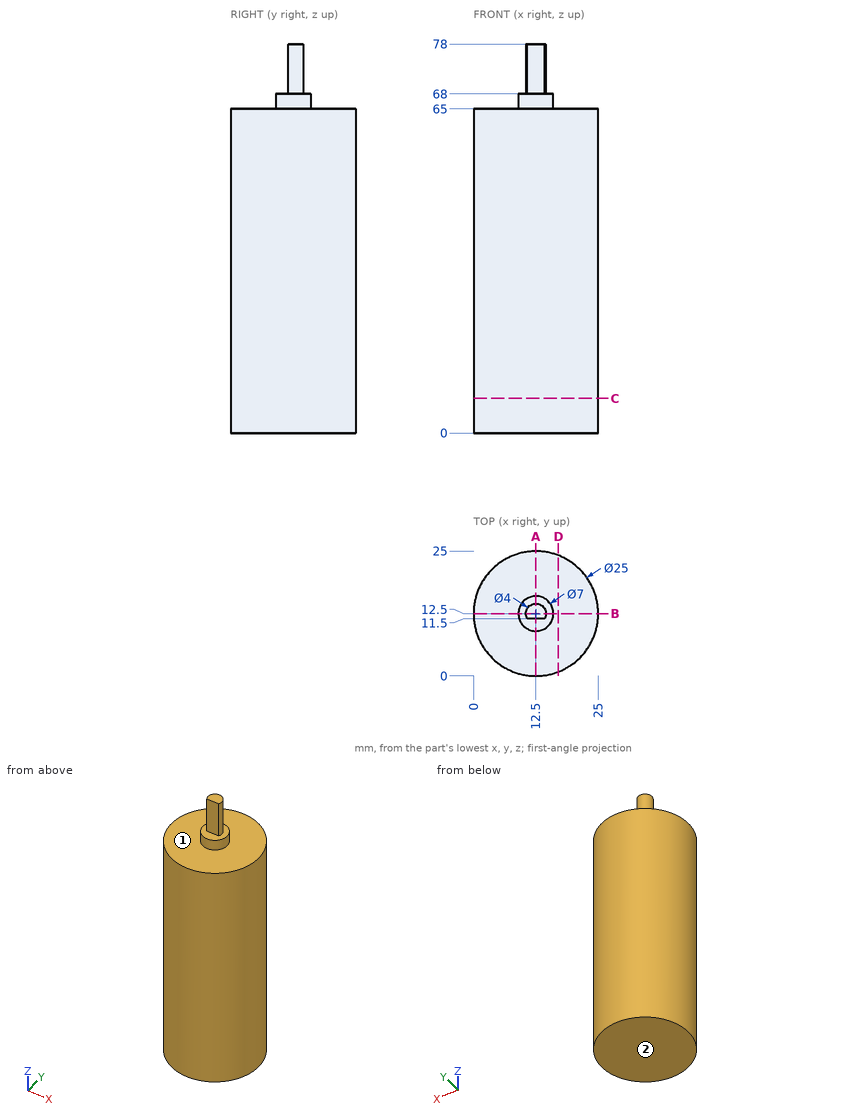
Answer from the drawing. Dimensions are ordinates in mm from the lowest x, y and z of the part. A direction names the side the tool comes from. Give positions to 0.01 mm unless a question says otherwise; leave off trailing zeros. Order: outer loops, then holes, each group sorted by start corner. A loop starts at its lowest first (then second) coordinate and runs counter-clockwise, first axis right, second up.
(1) Given pin 1 (1 mm diameter, centred on x = 13, z = 75.5, fed in from -Y); pin 2 (1.5 mm diameter, centred on y = 14, z = 22, fed in from -X); pin 3 (1 mm diameter, centred on x = 20.5, y = 3.5, fed in from +Z), each flat-ended and moving along its own axis, determine where each tip first touches the part or whether it passes through.
(2) For the marked faces 1 and 2, determine the directions among +Z, -Z, +X, -X, +Y, -Y from which every point of the face is accessible in a straight line to the end or side of a thin tool.
(3) Find section A-A (x = 12.5). Give the vertices of the cut face in (y, z).
(4) Find section B-B (y = 12.5). Give the vertices of the cut face in (x, z), plus the area to 3 significant figures.
(5) Find section C-C (z = 7). Give the vertices of the cut face in (x, y), plus the area to 3 significant figures.
(6) Straight lines are drawn through the part: L1, parallel to Z at x = 12, y = 23.25; L2, parallel to Y at x = 12, z = 45.5; L3, parallel to X at y = 3.5, z = 28.5 (1 decimal). For each, find the intervals that lie inside material, in ascending order.
(7) Find section D-D (x = 17). Give the vertices of the cut face in (y, z).
Result sheet:
1. pin 1: stops at y = 11.5
1. pin 2: stops at x = 0.02
1. pin 3: stops at z = 65
2. face 1: +Z
2. face 2: -Z, +X, -X, +Y, -Y
3. outline: (0, 0) - (25, 0) - (25, 65) - (16, 65) - (16, 68) - (14.5, 68) - (14.5, 78) - (11.5, 78) - (11.5, 68) - (9, 68) - (9, 65) - (0, 65) - close
4. outline: (0, 0) - (25, 0) - (25, 65) - (16, 65) - (16, 68) - (14.5, 68) - (14.5, 78) - (10.5, 78) - (10.5, 68) - (9, 68) - (9, 65) - (0, 65) - close
4. area: 1,690 mm2
5. outline: circle Ø25 at (12.5, 12.5)
5. area: 491 mm2
6. L1: z = 0 to 65
6. L2: y = 0.01 to 24.99
6. L3: x = 3.8 to 21.2
7. outline: (0.84, 0) - (24.16, 0) - (24.16, 65) - (0.84, 65) - close
